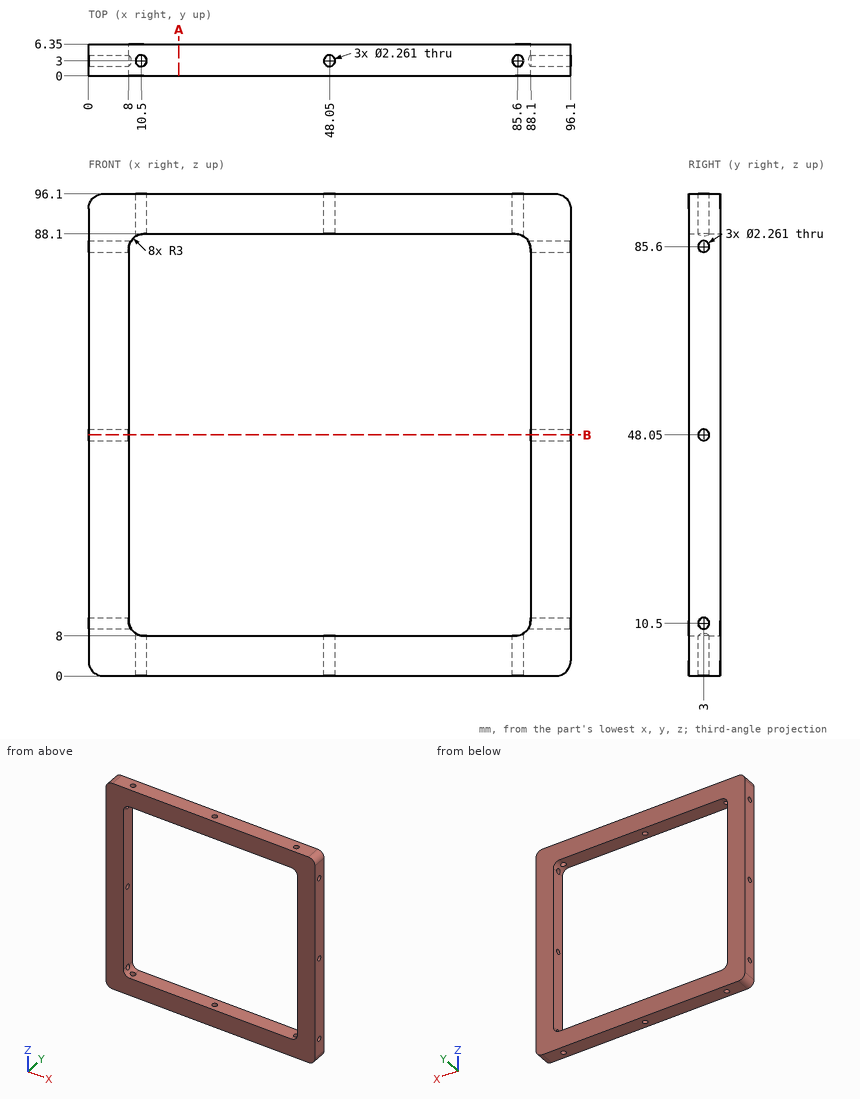
Print and shaded views of the part. All mm, measured from the part's lowest x, y and z. Give positions to 0.01 mm unless a question says otherwise; leave off trailing zeros. Order: outer loops, then holes, each group sorted by start corner. A loop starts at its lowest first (then second) coordinate and runs counter-clockwise, first axis right, second up. Notation, with made-up numbers: (2, 54.5) - (20, 54.5) arc R18 cw to (20, 62.5) - close; hole circle Ø4 at (35.25, 3.5). An arc over 180 degrees is marked (long way). Use a Markdown table: item, result.
1) Probe L1, parallel to Z at x = 52, y = 1.25; L2, parallel to Y at x = 85.6, z = 90. List the from-to ranges inside material, lowest first. Write a range as from..to.
Checked values:
| item | result |
|---|---|
| L1 | 0..8, 88.1..96.1 |
| L2 | 0..1.87, 4.13..6.35 |
2) Saw through at B-B on z = 48.05. List the corners of the cut face in (x, y).
Checked values:
| item | result |
|---|---|
| outline | (0, 0) - (8, 0) - (8, 1.87) - (0, 1.87) - close; (0, 4.13) - (8, 4.13) - (8, 6.35) - (0, 6.35) - close; (88.1, 0) - (96.1, 0) - (96.1, 1.87) - (88.1, 1.87) - close; (88.1, 4.13) - (96.1, 4.13) - (96.1, 6.35) - (88.1, 6.35) - close |
3) Flat gauge pin, fed straight in: P1, Ø2.5, axis at x = 48.05, y = 3, coming from the -Z side. Where does the tip first touch, or does it go through?
Checked values:
| item | result |
|---|---|
| P1 | z = 0 |
4) Saw through at A-A on x = 18. List the corners of the cut face in (y, z).
Checked values:
| item | result |
|---|---|
| outline | (0, 0) - (6.35, 0) - (6.35, 8) - (0, 8) - close; (0, 88.1) - (6.35, 88.1) - (6.35, 96.1) - (0, 96.1) - close |
